Check sheet for the drawn part. Datum: minimum x, y, z corner. Units: mm. A direction names the side the tool comes from. Give positions to 0.01 mm unless a question says otherwise; leave off trailing zeros. Write each loop counter-clockwise with the first axis right and the second up, starting at its lowest first coordinate (ties: lowest second). Pieces come first, ordered by that corner, then holes. Notation, with made-up numbers: (10, 24.25) -> (53, 24.25) arc R36 ccw to (53, 59.25) -> close; hole circle Ø3 at (55, -28.75). An arc over 180 degrees is marked (long way). Write item = value, one per line. Start each with the question number.
1. Mould release check, pull along X, two halves, no side actions. Record for the marked faces 1, 2 and 3: pulls with the +X half, pulls with the -X half, needs draft (parallel to the pull), parting line crosses it, or undercut.
2. Thickness scan on line 1 along X through (y, z) = (17.25, 9); line 2 along Y through (x, z) = (1.1, 15); line 3 along Z through (x, y) = (12.75, 1). Record the ranges inside material, lowest first.
3. Set-up check for the marked faces 4 and 5: record each of +Z, -Z, +X, -X, +Y, -Y from which the full face is reachable in a straight line by a thin tool's end or side.
4. Cross-section at D-D, the plane z = 5. Record the cut outline in (x, y).
5. Depth check by flat-ended pin: P1, Ø1.5, axis at x = 20.5, z = 16, coming from the +Y side; P2, Ø2.5, axis at y = 13, z = 15, coming from the +X side. Enter the tip coordinate at first touch or a pass-through.
6. Cross-section at B-B, the plane y = 9. Record the cut outline in (x, z).
7. Cross-section at C-C, the plane z = 10. Record the cut outline in (x, y).
8. Cross-section at A-A, the plane x = 14.5. Record the cut outline in (y, z).
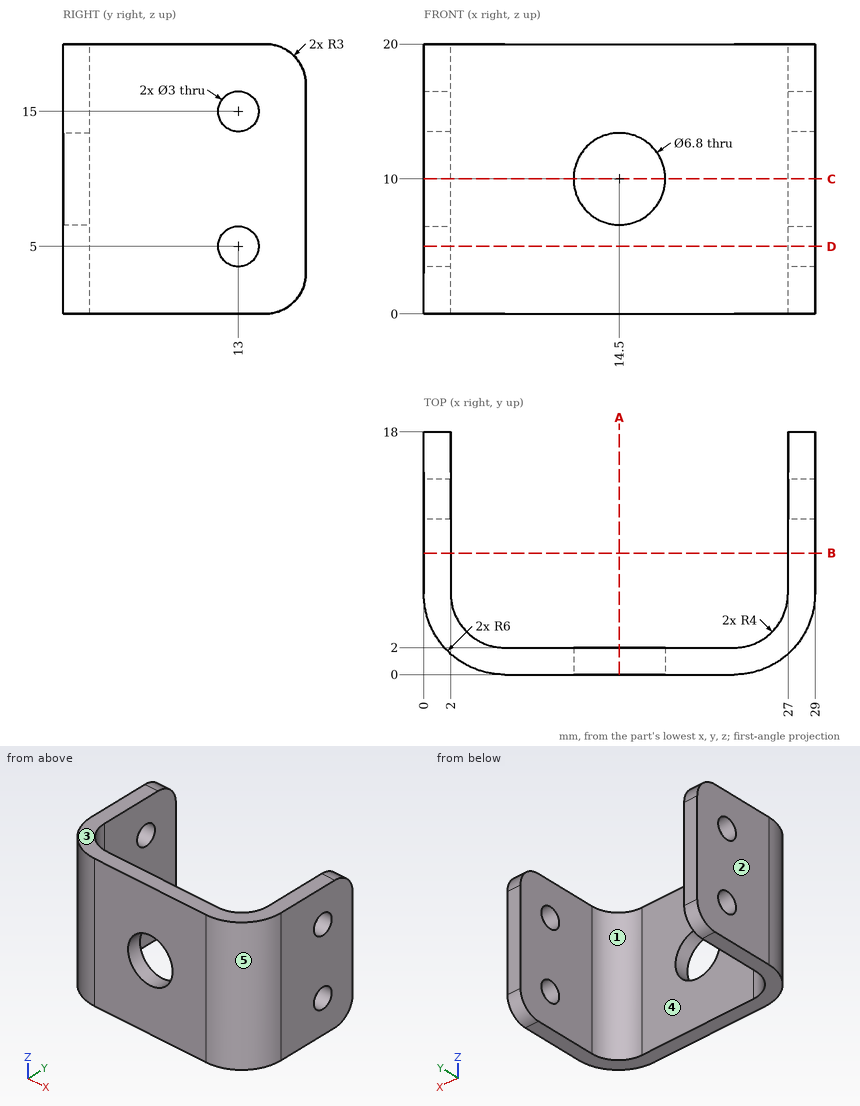
Answers:
q1.face_1 = undercut
q1.face_2 = pulls with the -X half
q1.face_3 = needs draft
q2.line_1 = 0 to 2, 27 to 29
q2.line_2 = 2.54 to 11.5, 14.5 to 18
q2.line_3 = 0 to 7.08, 12.92 to 20
q3.face_4 = +Z, -Z, +Y
q3.face_5 = +Z, -Z, +X, -Y
q4.outline = (0, 6) arc R6 ccw to (6, 0) -> (23, 0) arc R6 ccw to (29, 6) -> (29, 11.5) -> (27, 11.5) -> (27, 6) arc R4 cw to (23, 2) -> (6, 2) arc R4 cw to (2, 6) -> (2, 11.5) -> (0, 11.5) -> close; (0, 14.5) -> (2, 14.5) -> (2, 18) -> (0, 18) -> close; (27, 14.5) -> (29, 14.5) -> (29, 18) -> (27, 18) -> close
q5.P1 = 2
q5.P2 = through
q6.outline = (0, 0) -> (2, 0) -> (2, 20) -> (0, 20) -> close; (27, 0) -> (29, 0) -> (29, 20) -> (27, 20) -> close
q7.outline = (0, 6) arc R6 ccw to (6, 0) -> (11.1, 0) -> (11.1, 2) -> (6, 2) arc R4 cw to (2, 6) -> (2, 18) -> (0, 18) -> close; (17.9, 0) -> (23, 0) arc R6 ccw to (29, 6) -> (29, 18) -> (27, 18) -> (27, 6) arc R4 cw to (23, 2) -> (17.9, 2) -> close
q8.outline = (0, 0) -> (2, 0) -> (2, 6.6) -> (0, 6.6) -> close; (0, 13.4) -> (2, 13.4) -> (2, 20) -> (0, 20) -> close
